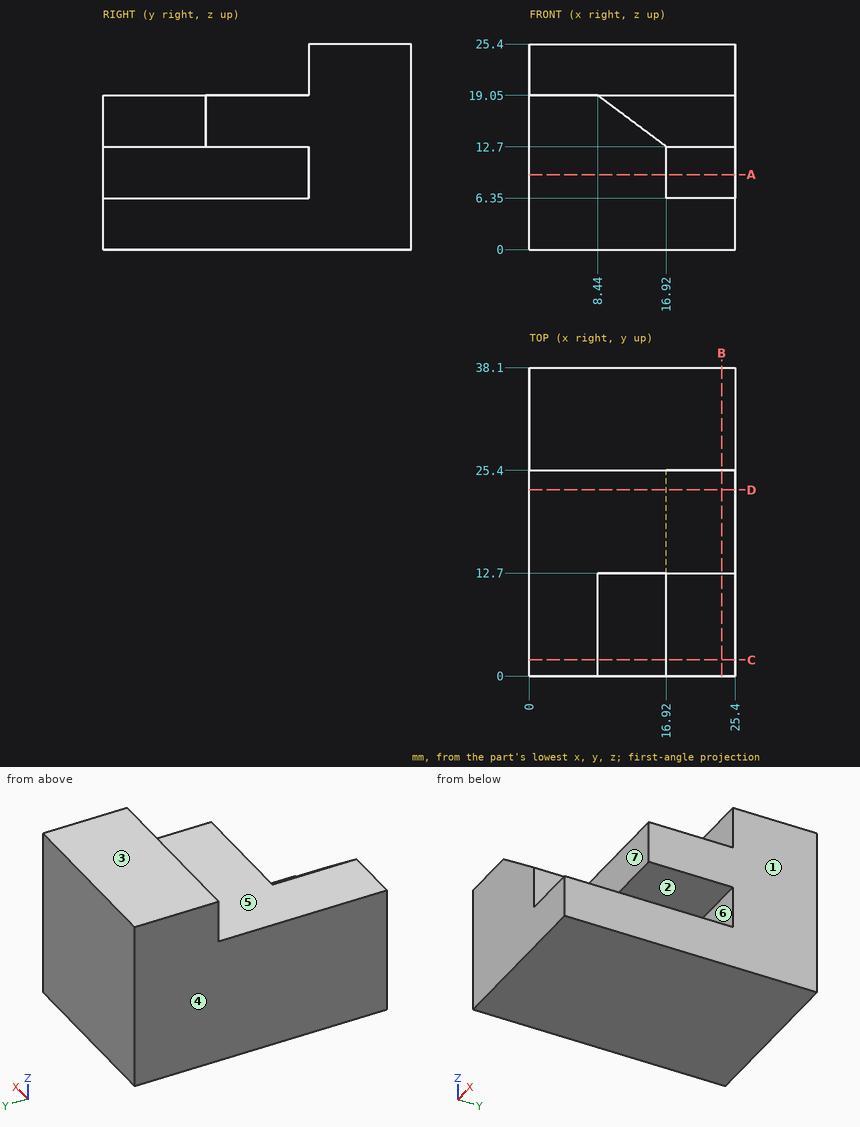
Source: three-view drawing plus pictorial views. Frame: mm from the lowest corner of the part. A direction names the side the tool comes from. Coordinates: 2 decimals unless noted, no trailing zeros. Loops run counter-clockwise (first coordinate to the right, second up) from the corner with the lowest first, then second, coordinate; pieces in that order, holes last. Notation, with made-up numbers: (34.5, -22) - (55.5, -22) arc R27 ccw to (55.5, 4) - close; hole circle Ø4 at (82.25, 54.5). An arc over 180 degrees is marked (long way). One line per question, with ' | ' between items.
1) Set-up query: the marked faces 4, 5, 6 and 7. Return all of +Z, -Z, +X, -X, +Y, -Y with unobstructed straight access to the full face (end or side cutting, diameter ignored); none if empty.
Report:
face 4: +Z, -Z, -X, +Y, -Y | face 5: +Z, +X, -X, -Y | face 6: +X, -Y | face 7: +Z, +X, -Y
2) First-contact query: P1, Ø12, axis at x = 21, z = 21.5, coming from the -Y side; P2, Ø1.5, axis at x = 19.5, y = 19, coming from the +Z side; P3, Ø1.9, axis at x = 16.5, z = 23, coming from the -Y side. Flat tips, straight axial feed; report the tip coordinate or a pass-through.
Report:
P1: stops at y = 12.7 | P2: stops at z = 19.05 | P3: stops at y = 25.4
3) Section A-A, the plane z = 9.25. Return loops of the section in (x, y).
Report:
outline: (0, 0) - (16.92, 0) - (16.92, 25.4) - (25.4, 25.4) - (25.4, 38.1) - (0, 38.1) - close
4) Section C-C, the plane y = 2. Return loops of the section in (x, z), then the cut area to 3 significant figures.
Report:
outline: (0, 0) - (25.4, 0) - (25.4, 6.35) - (16.92, 6.35) - (16.92, 12.7) - (8.44, 19.05) - (0, 19.05) - close | area: 349 mm²
5) Section B-B, the plane x = 23.75. Return loops of the section in (y, z).
Report:
outline: (0, 0) - (38.1, 0) - (38.1, 25.4) - (25.4, 25.4) - (25.4, 19.05) - (12.7, 19.05) - (12.7, 12.7) - (25.4, 12.7) - (25.4, 6.35) - (0, 6.35) - close
6) Line query: line 1 along Z through (x, y) = (20.75, 14); line 2 along Z through (x, y) = (20.25, 4.5); line 3 along Y through (x, z) = (2, 23.5). Output: solid intervals per line, ascending.
Report:
line 1: z = 0 to 6.35, 12.7 to 19.05 | line 2: z = 0 to 6.35 | line 3: y = 25.4 to 38.1
7) Section D-D, the plane y = 23. Return loops of the section in (x, z).
Report:
outline: (0, 0) - (25.4, 0) - (25.4, 6.35) - (16.92, 6.35) - (16.92, 12.7) - (25.4, 12.7) - (25.4, 19.05) - (0, 19.05) - close
8) Pull-direction query (Z, two-part tool) for the marked faces 1, 2 and 3; classes: released by +Z, released by -Z, zero draft, split by the parting line, or undercut.
Report:
face 1: zero draft | face 2: undercut | face 3: released by +Z
